Work out the finished part from the listing and answer in its coordinate system (mm). A direction names the side the tool comes from. Round coordinates to 2 decimals unless told otherwise and drop trailing zeros. Write each loop counter-clockwise with the first axis right and the second up, starting at its lowest first coordinate (ties: lowest second). Pieces come first, ordered by that corner, then holes.
1. Straight lines are drawn through the part: probe 1 along Y at (x, z) = (1.5, -2); probe 2 along X at (y, z) = (-2.5, 1); probe 3 along X at (y, z) = (0, -4.5). For each, find the intervals that lie inside material, in ascending order.
2. A tool of negligible diameter and unlimited length cuts with its end or side. For faces 4 (the face through (4.2, 0.1, -3.3)), 5 (the face through (1.732, 0.985, 0.971)), from which of +Z, -Z, +X, -X, +Y, -Y can it reach the whole face along a straight path? Write none if from no direction.
3. Find section C-C (y = 4.25). Write down the section's boundary in (x, z), and give its area (3 significant figures).
4. Find section B-B (z = 3.25). Write down the section's boundary in (x, y), and give its area (3 significant figures).
5. Find section A-A (x = 22). Write down the section's boundary in (y, z), and give its area (3 significant figures).
6. Flat-ended cylindrical pins translate along their axes: pin 1 Ø3 at (x, z) = (16, 0.5) entering from +Y; pin 2 Ø0.6 at (y, z) = (0, 1.5) entering from -X; pin 3 Ø2 at (x, z) = (17, 2) entering from -Y. Find the tip coordinate at first contact, or state that the pin passes through.
7. Determine the mould class of faces 1 (the face through (24.2, 0, 0)), 2 (the face through (14, -3, 0)), 3 (the face through (2.11, -2.45, 0.01)) for opening direction Z: pulls with the +Z half, pulls with the -Z half, needs draft (parallel to the pull), parting line crosses it, or undercut.
```python
from build123d import *

# Parameters (mm, degrees)
SKETCH3_W    = 0.82
SKETCH3_H    = 7
SKETCH4_W    = 0.82
SKETCH4_H    = 3.809077818
RECPAT_COUNT = 2
RECPAT_ANGLE = 90


with BuildPart() as part:
    # BodySke → Base-Revolve (revolve)
    with BuildSketch(Plane.XY):
        with BuildLine():
            Line((4.2, 3), (4.2, 5.019960159))
            ThreePointArc((4.2, 5.019960159), (1.188478557, 3.272613634), (0, 0))
            Line((0, 0), (24.2, 0))
            Line((24.2, 0), (24.2, 3))
            Line((24.2, 3), (4.2, 3))
        make_face()
    revolve(axis=Axis((-25.4, 0, 0), (1, 0, 0)))

    # Sketch3 → Recess section 0
    with BuildSketch(Plane(origin=(0, 0, 0), x_dir=(0, 0, -1), z_dir=(1, 0, 0))):
        Rectangle(SKETCH3_W, SKETCH3_H)
    # Sketch4 → Recess section 1
    with BuildSketch(Plane(origin=(3.2, 0, 0), x_dir=(0, 0, -1), z_dir=(1, 0, 0))):
        Rectangle(SKETCH4_W, SKETCH4_H)
    recess = loft(mode=Mode.SUBTRACT)

    # RecPat: Recess ×2 about axis
    recpat_axis = Axis((0, 0, 0), (1, 0, 0))
    for i in range(1, RECPAT_COUNT):
        add(recess.rotate(recpat_axis, i * RECPAT_ANGLE / (RECPAT_COUNT - 1)), mode=Mode.SUBTRACT)

    # RecCorSke → RecessCore (revolve, cut)
    with BuildSketch(Plane.XY):
        Polygon((0, 0), (0, 1.504265798), (3.2, 1.2805), (3.616059671, 0), align=None)
    revolve(axis=Axis((-3.175, 0, 0), (1, 0, 0)), mode=Mode.SUBTRACT)


solid = part.part
```
Worked answers:
1. probe 1: y = -3.01 to -0.41, 0.41 to 3.01
1. probe 2: x = 0.77 to 24.2
1. probe 3: x = 2.7 to 4.2
2. face 4: +X
2. face 5: -X
3. outline: (4.2, -2.67) - (4.2, 2.67) arc R2.82 ccw to start
3. area: 7.50 mm2
4. outline: (4.2, -3.83) - (4.2, 3.83) arc R3.93 ccw to start
4. area: 17.3 mm2
5. outline: circle Ø6 at (0, 0)
5. area: 28.3 mm2
6. pin 1: stops at y = 3
6. pin 2: stops at x = 3.2
6. pin 3: stops at y = -2.83
7. face 1: needs draft
7. face 2: parting line crosses it
7. face 3: undercut
